Part model, mm, in its own coordinate system. A direction names the side the tool comes from. Coordinates: 2 decimals unless noted, no trailing zeros. Order: outer loops, then holes, each group sorted by start corner. A loop starts at its lowest first (then second) coordinate and runs counter-clockwise, first axis right, second up.
1) Cut at D-D (z = 2.5). List the corners of the cut face in (x, y).
2) Cut at C-C (z = -6.25). List the corners of the cut face in (x, y).
3) Tool access for faces 1 (the flat face through (41, -15.623, -4)), 2 (the flat face through (4, -13, -4.616)), 3 (the flat face through (43.679, -13, -7)): list every direction of +Z, -Z, +X, -X, +Y, -Y with a clear straight run to the whole face (end or side of a thin tool).
4) Cut at B-B (y = -14.5). List the corners of the cut face in (x, z), and give its area (3 significant figures).
5) Wall check: L1, parallel to X at y = -15, z = -6; L2, parallel to Y at x = 40, z = -1.75; L3, parallel to Z at x = 76.5, y = -16. Give the ranges that are in metal, low to high.
6) Mould opens along Y. For faces 4 (the flat face through (41, -20.121, -5)), 5 (the flat face through (35.158, -13, -7)), 6 (the flat face through (41, -9, 11.836)) say: +Y half, -Y half, draft (parallel to the pull), parting line (faces both ways), or undercut.
7) Pin check, flat tips, straight feed: pin 1 Ø1.4 at (x, y) = (76.5, -12.5) entering from +Z; pin 2 Ø5 at (x, y) = (54, -18.5) entering from +Z. Stop position of each tip, or through.
8) Cut at A-A (x = 38.5). List the corners of the cut face in (y, z), and give its area (3 significant figures).
```python
from build123d import *

# Parameters (mm, degrees)
F0_W     = 4.4976044446
F0_H     = 4.615961574
F0_W_2   = 4.7343205661
F1_DEPTH = 83.312
F2_W     = 8.285057731
F2_H     = 4.7343205661
F2_W_2   = 8.5217729211
F2_W_3   = 6.1546228826
F3_DEPTH = 27.94


with BuildPart() as f1:
    # F0 (on Right) → F1 (new body)
    with BuildSketch(Plane.YZ):
        with Locations((-17.8720569238, -6.923942361)):
            Rectangle(F0_W, F0_H)
        with Locations((-13.2560944185, -6.923942361)):
            Rectangle(F0_W_2, F0_H)
        with Locations((-17.8720569238, -2.307980787)):
            Rectangle(F0_W, F0_H)
        Polygon((-10.8889341354, -4.615961574), (-10.8889341354, -9.231923148), (-6.6280476749, -9.231923148), (-6.6280476749, 11.8357995525), (-10.8889341354, 11.8357995525), align=None)
    extrude(amount=F1_DEPTH)

    # F2 (on face) → F3 (cut)
    with BuildSketch(Plane.XY.offset(-4.615961574)):
        with Locations((13.0246370099, -13.2560944185)):
            Rectangle(F2_W, F2_H)
        with Locations((39.4184701145, -13.2560944185)):
            Rectangle(F2_W_2, F2_H)
        with Locations((64.0369299799, -13.2560944185)):
            Rectangle(F2_W_3, F2_H)
    extrude(amount=-F3_DEPTH, mode=Mode.SUBTRACT)


solid = f1.part
```
Geometry check:
1. outline: (0, -10.89) - (83.31, -10.89) - (83.31, -6.63) - (0, -6.63) - close
2. outline: (0, -20.12) - (83.31, -20.12) - (83.31, -6.63) - (0, -6.63) - close; hole (8.88, -15.62) - (17.17, -15.62) - (17.17, -10.89) - (8.88, -10.89) - close; hole (35.16, -15.62) - (43.68, -15.62) - (43.68, -10.89) - (35.16, -10.89) - close; hole (60.96, -15.62) - (67.11, -15.62) - (67.11, -10.89) - (60.96, -10.89) - close
3. face 1: +Z
3. face 2: +Z, +X, -X
3. face 3: +Z, -Z
4. outline: (0, -9.23) - (8.88, -9.23) - (8.88, -4.62) - (0, -4.62) - close; (17.17, -9.23) - (35.16, -9.23) - (35.16, -4.62) - (17.17, -4.62) - close; (43.68, -9.23) - (60.96, -9.23) - (60.96, -4.62) - (43.68, -4.62) - close; (67.11, -9.23) - (83.31, -9.23) - (83.31, -4.62) - (67.11, -4.62) - close
4. area: 279 mm2
5. L1: x = 0 to 8.88, 17.17 to 35.16, 43.68 to 60.96, 67.11 to 83.31
5. L2: y = -20.12 to -15.62, -10.89 to -6.63
5. L3: z = -9.23 to 0
6. face 4: -Y half
6. face 5: undercut
6. face 6: draft
7. pin 1: stops at z = -4.62
7. pin 2: stops at z = 0
8. outline: (-20.12, -9.23) - (-15.62, -9.23) - (-15.62, 0) - (-20.12, 0) - close; (-10.89, -9.23) - (-6.63, -9.23) - (-6.63, 11.84) - (-10.89, 11.84) - close
8. area: 131 mm2
